Drawing for the job (mm, zero at the part's lowest x, y, z). A direction names the side the tool comes from. Round coordinates to 2 decimals unless told otherwise and drop trailing zeros. Write each loop counter-clockwise with the first axis right and the second up, starting at its lowest first coordinate (ties: lowest second). Pieces come first, ordered by that corner, then holes. Notation, with made-up numbers: M 9,80.5 L 23,80.5 A16 ccw 23,87.5 Z; hole C 88.25,22 d10. An arc over 180 degrees is marked long. Use a Markdown table: item, result. Add a question column.
1) Slice it at B-B on x = 68. Write the cut outline in (y, z).
2) Which spindle directions (+Z, -Z, +X, -X, +Y, -Y) get a long thin tool onto all of the face, cutting with end or side? Do the marked faces 1, 2 and 3. Say none if no direction does.
3) Slice it at D-D on z = 92. Write the cut outline in (x, y) (1 decimal).
4) Slice it at A-A on z = 51. Write the cut outline in (x, y) (1 decimal), plus the area to 3 significant figures.
5) Drop flat-ended pins along their axis: P1, Ø6, axis at y = 34, z = 106.5, coming from the -X side (1 decimal); P2, Ø2, axis at y = 10, z = 33, coming from the -X side; P3, Ø12, axis at x = 99, y = 24.5, coming from the +Z side. Give the stop position or say it passes through.
6) Wall check: probe 1 along Y at (x, z) = (106.5, 97.5); probe 2 along X at (y, z) = (30, 64); probe 3 along X at (y, z) = (31, 78.5) (1 decimal). Give the ranges that are in metal, low to high.
7) Slice it at C-C on y = 38. Write the cut outline in (x, z) (1 decimal), plus the area to 3 significant figures.
8) Two-plate mould, pull along X, no slides. Class the marked faces 4, 5 and 6: released by +X, released by -X, zero draft, split by the parting line, or undercut.
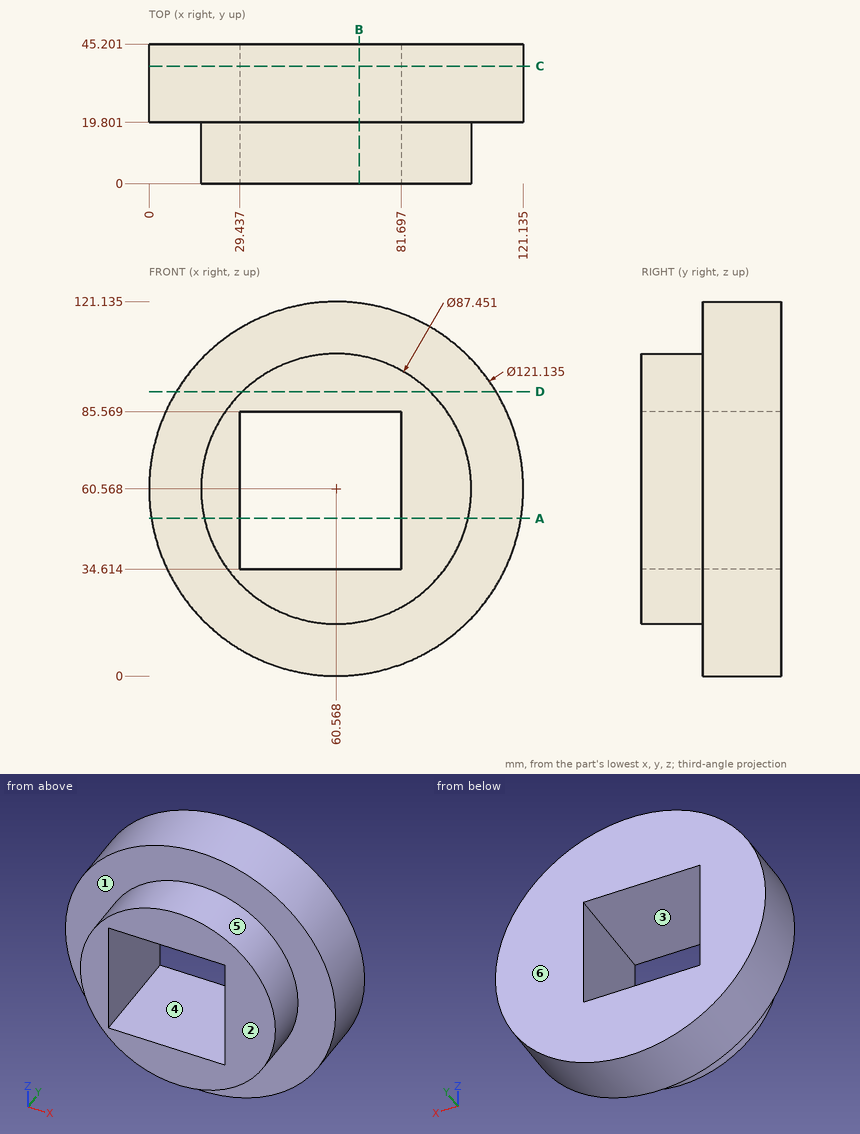
Entries:
| question | item | result |
|---|---|---|
| 1 | outline | M 0,17.48 L 19.8,17.48 L 19.8,0.46 L 45.2,0.46 L 45.2,34.61 L 0,34.61 Z; M 0,85.57 L 45.2,85.57 L 45.2,120.68 L 19.8,120.68 L 19.8,103.66 L 0,103.66 Z |
| 2 | face 1 | -Y |
| 2 | face 2 | +Z, -Z, +X, -X, -Y |
| 2 | face 3 | +Y, -Y |
| 3 | outline | M 8.8,19.8 L 30.2,19.8 L 30.2,0 L 91,0 L 91,19.8 L 112.3,19.8 L 112.3,45.2 L 8.8,45.2 Z |
| 4 | outline | M 0.8,19.8 L 17.9,19.8 L 17.9,0 L 29.4,0 L 29.4,45.2 L 0.8,45.2 Z; M 81.7,0 L 103.2,0 L 103.2,19.8 L 120.4,19.8 L 120.4,45.2 L 81.7,45.2 Z |
| 4 | area | 2,370 mm^2 |
| 5 | P1 | stops at x = 17.8 |
| 5 | P2 | stops at x = 25.84 |
| 5 | P3 | stops at z = 111.72 |
| 6 | probe 1 | y = 19.8 to 45.2 |
| 6 | probe 2 | x = 0.1 to 29.44, 81.7 to 121.04 |
| 6 | probe 3 | x = 2.7 to 29.4, 81.7 to 118.4 |
| 7 | outline | C 60.6,60.6 d121.1; hole M 29.4,34.6 L 81.7,34.6 L 81.7,85.6 L 29.4,85.6 Z |
| 7 | area | 8,860 mm^2 |
| 8 | face 4 | undercut |
| 8 | face 5 | split by the parting line |
| 8 | face 6 | zero draft |
